Can you work these out from the model? Positions are in its coordinate system, mm. A direction names the side the tool comes from. Give positions to 0.01 mm unless a question says otherwise; leave off trailing zeros. Loops run counter-clockwise (first coordinate to the right, second up) from the corner with the lowest first, then second, coordinate; pieces in that order, holes last. Notation, with made-up numbers: (4, 25) - (21, 25) arc R13 cw to (21, 31) - close; hole circle Ø4 at (21, -26.75). An arc over 180 degrees is marked (long way). Answer as a JSON object with one key per item and string values. Group by question number.
Item 1: Will these pins go through, and if not, where does the flat tip stop? pin 1 (4 mm diameter, centred on y = 5, z = 14.5, fed in from +X); pin 2 (8 mm diameter, centred on y = 12, z = -37, fed in from -X); pin 3 (4 mm diameter, centred on x = 10, z = 35, fed in from +Y).
Item 2: Please list where these lines run through material, in increasing order: L1, parallel to X at y = 0.85, z = 35; L2, parallel to Z at x = 0.5, y = 10.5.
Item 3: Which directions (+Z, -Z, +X, -X, +Y, -Y) give clear straight access to the entire face, cutting with the end or side of a thin tool? Please do faces 1 (the cylindrical face through (0.8, 9.1, 1.2)), 2 (the flat face through (8, 1.5, -1)).
Item 4: Suppose I cut it at A-A on y = 10. Write out the boundary of the cut face in (x, z).
Item 5: Suppose I cut it at B-B on z = 0. Write out the boundary of the cut face in (x, y).
Item 6: Thinking about a two-plate mould opening in Z: for faces 3 (the flat face through (4, 1, 75)), 4 (the cylindrical face through (9.1, 0.7, -33.8)), 5 (the flat face through (1.5, 8, -1)), which applies, pulls with the +Z half, pulls with the -Z half, needs draft (parallel to the pull), parting line crosses it, or undercut?
Item 7: Suppose I cut it at C-C on x = 13. Write out the boundary of the cut face in (y, z).
from build123d import *

# Parameters (mm, degrees)
EXTRUSION1_DEPTH           = 75
EXTRUSION1_DEPTH_BACK      = 75
ESQUISSE2_R                = 1.5
EXTRUSION2_DEPTH           = 78.667560796
ESQUISSE3_R                = 1.5
EXTRUSION3_DEPTH           = 78.942286341
R_P_TITION_LIN_AIRE1_COUNT = 3
R_P_TITION_LIN_AIRE1_PITCH = 50
R_P_TITION_LIN_AIRE2_COUNT = 5
R_P_TITION_LIN_AIRE2_PITCH = 35


with BuildPart() as part:
    # Esquisse1 → Extrusion1 (new, two sides: drawn at the far end of the back side and taken through both)
    with BuildSketch(Plane.XY.offset(-EXTRUSION1_DEPTH_BACK)):
        Polygon((0, 0), (2, 0), (15, 0), (15, 1.5), (1.5, 1.5), (1.5, 15), (0, 15), align=None)
    extrude(amount=EXTRUSION1_DEPTH + EXTRUSION1_DEPTH_BACK)

    # Esquisse2 → Extrusion2 (cut, through all)
    with BuildSketch(Plane(origin=(1.5, 0, 0), x_dir=(0, 0, -1), z_dir=(1, 0, 0))):
        with Locations((-50, 10)):
            Circle(ESQUISSE2_R)
    extrusion2 = extrude(amount=-EXTRUSION2_DEPTH, mode=Mode.SUBTRACT)

    # Esquisse3 → Extrusion3 (cut, through all)
    with BuildSketch(Plane.XZ):
        with Locations(Location((10, 70, 0), (0, 0, 270))):
            Circle(ESQUISSE3_R)
    extrusion3 = extrude(amount=-EXTRUSION3_DEPTH, mode=Mode.SUBTRACT)

    # R_p_tition lin_aire1: Extrusion2 ×3
    with Locations(*[(0, 0, -i * R_P_TITION_LIN_AIRE1_PITCH) for i in range(1, R_P_TITION_LIN_AIRE1_COUNT)]):
        add(extrusion2, mode=Mode.SUBTRACT)

    # R_p_tition lin_aire2: Extrusion3 ×5, 1 skipped
    with Locations(*[(0, 0, -i * R_P_TITION_LIN_AIRE2_PITCH) for i in range(1, R_P_TITION_LIN_AIRE2_COUNT) if i not in (2,)]):
        add(extrusion3, mode=Mode.SUBTRACT)


solid = part.part
Worked out:
{
 "1": {"pin 1": "stops at x = 1.5", "pin 2": "stops at x = 0", "pin 3": "stops at y = 1.5"},
 "2": {"L1": "x = 0 to 8.5, 11.5 to 15", "L2": "z = -75 to -51.41, -48.59 to -1.41, 1.41 to 48.59, 51.41 to 75"},
 "3": {"face 1": "+X, -X", "face 2": "+Z, -Z, +X, +Y"},
 "4": {"outline": "(0, -75) - (1.5, -75) - (1.5, -51.5) - (0, -51.5) - close; (0, -48.5) - (1.5, -48.5) - (1.5, -1.5) - (0, -1.5) - close; (0, 1.5) - (1.5, 1.5) - (1.5, 48.5) - (0, 48.5) - close; (0, 51.5) - (1.5, 51.5) - (1.5, 75) - (0, 75) - close"},
 "5": {"outline": "(0, 0) - (15, 0) - (15, 1.5) - (1.5, 1.5) - (1.5, 8.5) - (0, 8.5) - close; (0, 11.5) - (1.5, 11.5) - (1.5, 15) - (0, 15) - close"},
 "6": {"face 3": "pulls with the +Z half", "face 4": "undercut", "face 5": "needs draft"},
 "7": {"outline": "(0, -75) - (1.5, -75) - (1.5, 75) - (0, 75) - close"}
}
